Check sheet for the modelled part. Datum: model origin and axes. Units: mm. A direction names the side the tool comes from. Round coordinates to 2 decimals unless told otherwise and drop trailing zeros. Write each loop counter-clockwise with the first axis right and the second up, starting at its lowest first coordinate (ties: lowest second). Pieces come first, ordered by that corner, then holes. Notation, with made-up numbers: M 73,62.25 L 103,62.25 A27 cw 103,88.25 Z; hole C -27.5,-30.5 d3. An arc over 180 degrees is marked long. Put each result on its own line as item: value.
```python
from build123d import *

# Parameters (mm, degrees)
F0_R     = 12
F1_DEPTH = 25
F3_DEPTH = 25


with BuildPart() as f1:
    # F0 (on Right) → F1 (new body)
    with BuildSketch(Plane.YZ):
        with BuildLine():
            Line((15, -53.741885), (15, 25.757949))
            ThreePointArc((15, 25.757949), (-10.323708, 36.640093), (-0.789474, 10.778739))
            ThreePointArc((-0.789474, 10.778739), (1.901905, 9.537272), (3, 6.784283))
            Line((3, 6.784283), (3, -53.741885))
            Line((3, -53.741885), (15, -53.741885))
        make_face()
        with Locations((0, 25.757949)):
            Circle(F0_R, mode=Mode.SUBTRACT)
    extrude(amount=F1_DEPTH)

    # F2 (on face) → F3 (cut)
    with BuildSketch(Plane(origin=(0, 15, 0), x_dir=(-1, 0, 0), z_dir=(0, 1, 0))):
        with BuildLine():
            Line((0, -53.741885), (0, -41.241885))
            ThreePointArc((0, -41.241885), (-3.661165, -50.080719), (-12.5, -53.741885))
            Line((-12.5, -53.741885), (0, -53.741885))
        make_face()
        with BuildLine():
            Line((-25, -53.741885), (-12.5, -53.741885))
            ThreePointArc((-12.5, -53.741885), (-21.338835, -50.080719), (-25, -41.241885))
            Line((-25, -41.241885), (-25, -53.741885))
        make_face()
        with BuildLine():
            Line((-6.5, -41.241885), (-6.5, -19.129273))
            ThreePointArc((-6.5, -19.129273), (-12.5, -13.129273), (-18.5, -19.129273))
            Line((-18.5, -19.129273), (-18.5, -41.241885))
            ThreePointArc((-18.5, -41.241885), (-12.5, -47.241885), (-6.5, -41.241885))
        make_face()
    extrude(amount=-F3_DEPTH, mode=Mode.SUBTRACT)


solid = f1.part
```
1. Cross-section at D-D (y = 6.5). Enter the section's corners in (x, z), then the cut area to 3 significant figures.
Computed values:
outline: M 0,-41.24 A12.5 ccw 12.5,-53.74 A12.5 ccw 25,-41.24 L 25,15.67 L 0,15.67 Z; M 0,35.85 L 25,35.85 L 25,39.28 L 0,39.28 Z; hole M 6.5,-41.24 A6 ccw 18.5,-41.24 L 18.5,-19.13 A6 ccw 6.5,-19.13 Z
area: 1,380 mm2
2. Release check for a two-part mould opening along Z. For faces 4 (the cylindrical face through (12.37, 9.08, -13.13)), 5 (the cylindrical face through (12.325, -9.963, 36.971)), 6 (the flat face through (0, 6, 0)) record: +Z half, -Z half, draft (parallel to the pull), parting line (faces both ways), or undercut.
Computed values:
face 4: undercut
face 5: parting line
face 6: draft
3. Cross-section at A-A (x = 15.25). Enter the section's corners in (y, z).
Computed values:
outline: M -0.79,10.78 A4 cw 3,6.78 L 3,-13.8 L 15,-13.8 L 15,25.76 A15 ccw long Z; M 3,-53.44 L 15,-53.44 L 15,-46.57 L 3,-46.57 Z; hole C 0,25.76 d24
4. Depth check by flat-ended pin: pin 1 Ø12 at (x, y) = (19.5, -8.5) entering from +Z; pin 2 Ø6 at (x, y) = (6.5, 10.5) entering from +Z; pin 3 Ø12 at (y, z) = (-0.5, 24) entering from -X; pin 4 Ø5 at (y, z) = (1, 6) entering from +X. Enter the tip coordinate at first touch or a pass-through.
Computed values:
pin 1: stops at z = 40.55
pin 2: stops at z = 38.75
pin 3: passes through
pin 4: stops at x = 25
5. Cross-section at B-B (z = -39). Enter the section's corners in (x, y), then the cut area to 3 significant figures.
Computed values:
outline: M 0,3 L 6.5,3 L 6.5,15 L 0,15 Z; M 18.5,3 L 25,3 L 25,15 L 18.5,15 Z
area: 156 mm2
6. Scan lines: probe 1 along Y at (x, z) = (15.5, 4); probe 2 along Z at (x, y) = (23.5, 5); probe 3 along Z at (x, y) = (7.5, 12.5). Record each from-to range of solid material in increasing order.
Computed values:
probe 1: y = 3 to 15
probe 2: z = -47.18 to 14.85, 36.67 to 39.9
probe 3: z = -52.7 to -44.56, -15.81 to 34.05
7. Cross-section at C-C (y = -5). Enter the section's corners in (x, z), then the cut area to 3 significant figures.
Computed values:
outline: M 0,11.62 L 25,11.62 L 25,14.85 L 0,14.85 Z; M 0,36.67 L 25,36.67 L 25,39.9 L 0,39.9 Z
area: 162 mm2
8. Access from +Z, -Z, +X, -X, +Y, -Y to the whole of each face (thin tool, end or side, straight path). Record for faces 1 (the cylindrical face through (12.325, -2.601, 14.043)), 2 (the flat face through (6.5, 9, -30)), 3 (the flat face through (7, 3, -16)).
Computed values:
face 1: +X, -X
face 2: +Y, -Y
face 3: -Z, +X, -X, -Y
